Here's the drawing with two shaded views (mm, measured from the low corner). I have some questions. Coordinates: 2 decimals unless noted, no trailing zeros. Loops run counter-clockwise (first coordinate to the right, second up) from the corner with the lowest first, then second, coordinate; pieces in that order, holes last. Notation, with made-up numbers: (25.25, 85.5) -> (32.25, 85.5) arc R30 ccw to (32.25, 119.5) -> close; hole circle Ø2 at (-23.75, 41). An arc over 180 degrees is marked (long way). Answer as a JSON object with one key per item and string values. Group by question number.
1) I want a section at A-A (z = 2.35). Write out the boundary of the cut face in (x, y).
2) I want a section at B-B (y = 51). Write out the boundary of the cut face in (x, z) (3 decimals).
3) I need wall thicknesses on probe 1 along X at (y, z) = (72, 0.7); probe 2 along X at (y, z) = (64, 1). Which ranges of each line are inside material? Lowest first, please. Write a range as [from, to].
4) I'm going to push a flat-ended pin straight in: pin 1 (1 mm diameter, centred on y = 62, z = 2.5, fed in from +X). Where does the tip first touch, or does it pass through?
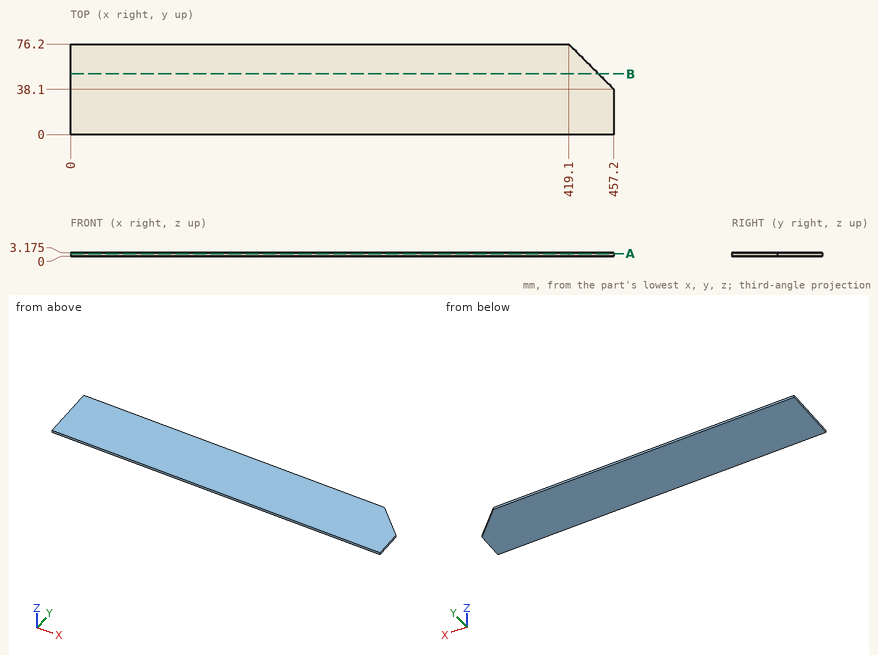
Determined:
{
 "1": {"outline": "(0, 0) -> (457.2, 0) -> (457.2, 38.1) -> (419.1, 76.2) -> (0, 76.2) -> close"},
 "2": {"outline": "(0, 0) -> (444.3, 0) -> (444.3, 3.175) -> (0, 3.175) -> close"},
 "3": {"probe 1": "[0, 423.3]", "probe 2": "[0, 431.3]"},
 "4": {"pin 1": "x = 433.8"}
}
